Read the model definition and answer for the solid it produces. Units are mm, in the model's axes. A direction names the side the tool comes from. Give positions to 0.01 mm unless a question says otherwise; leave off trailing zeros. Write each loop counter-clockwise with the first axis right and the second up, starting at its lowest first coordinate (ties: lowest second). Pieces come first, ordered by that corner, then holes. Notation, with made-up numbers: M 81.25,25 L 127.25,25 A8 cw 127.25,38 Z; hole C -30.5,14.5 d7. An arc over 180 degrees is marked long. Put each result on its own line as item: value.
from build123d import *

# Parameters (mm, degrees)
SKETCH1_W           = 25.4
SKETCH1_H           = 19.05
SKETCH1_R           = 3.175
SKETCH1_R_2         = 1.016
BOSS_EXTRUDE1_DEPTH = 5
SKETCH1_3_W         = 25.4
SKETCH1_3_H         = 5
BOSS_EXTRUDE2_DEPTH = 20
BOSS_EXTRUDE3_START = 20
SKETCH1_4_W         = 25.4
SKETCH1_4_H         = 19.05
SKETCH1_4_R         = 3.175
SKETCH1_4_R_2       = 1.016
BOSS_EXTRUDE3_DEPTH = 5
SKETCH2_R           = 1.0922
CUT_EXTRUDE1_DEPTH  = 10


with BuildPart() as part:
    # Sketch1 → Boss-Extrude1 (new body)
    with BuildSketch(Plane.XY):
        with Locations((12.7, -9.525)):
            Rectangle(SKETCH1_W, SKETCH1_H)
        with Locations((12.7, -9.525)):
            Circle(SKETCH1_R, mode=Mode.SUBTRACT)
        with Locations((17.4498, -14.2748)):
            Circle(SKETCH1_R_2, mode=Mode.SUBTRACT)
        with Locations((7.9502, -14.2748)):
            Circle(SKETCH1_R_2, mode=Mode.SUBTRACT)
        with Locations((17.4498, -4.7752)):
            Circle(SKETCH1_R_2, mode=Mode.SUBTRACT)
        with Locations((7.9502, -4.7752)):
            Circle(SKETCH1_R_2, mode=Mode.SUBTRACT)
    extrude(amount=BOSS_EXTRUDE1_DEPTH)

    # Sketch1<3> → Boss-Extrude2 (add)
    with BuildSketch(Plane.XY):
        with Locations((12.7, -21.55)):
            Rectangle(SKETCH1_3_W, SKETCH1_3_H)
        Polygon((30.4, 0), (30.4, -24.05), (25.4, -24.05), (25.4, -19.05), (25.4, 0), align=None)
        Polygon((-5, 0), (-5, -24.05), (0, -24.05), (0, -19.05), (0, 0), align=None)
    extrude(amount=BOSS_EXTRUDE2_DEPTH)

    # Sketch1<4> → Boss-Extrude3 (add)
    with BuildSketch(Plane.XY.offset(BOSS_EXTRUDE3_START)):
        with Locations((12.7, -9.525)):
            Rectangle(SKETCH1_4_W, SKETCH1_4_H)
        with Locations((12.7, -9.525)):
            Circle(SKETCH1_4_R, mode=Mode.SUBTRACT)
        with Locations((17.4498, -14.2748)):
            Circle(SKETCH1_4_R_2, mode=Mode.SUBTRACT)
        with Locations((7.9502, -14.2748)):
            Circle(SKETCH1_4_R_2, mode=Mode.SUBTRACT)
        with Locations((17.4498, -4.7752)):
            Circle(SKETCH1_4_R_2, mode=Mode.SUBTRACT)
        with Locations((7.9502, -4.7752)):
            Circle(SKETCH1_4_R_2, mode=Mode.SUBTRACT)
    extrude(amount=-BOSS_EXTRUDE3_DEPTH)

    # Sketch2 → Cut-Extrude1 (cut)
    with BuildSketch(Plane(origin=(0, 0, 0), x_dir=(1, 0, 0), z_dir=(0, 1, 0))):
        with Locations((-2.5, -2.5)):
            Circle(SKETCH2_R)
        with Locations((27.9, -2.5)):
            Circle(SKETCH2_R)
        with Locations((27.9, -17.5)):
            Circle(SKETCH2_R)
        with Locations((-2.5, -17.5)):
            Circle(SKETCH2_R)
    extrude(amount=-CUT_EXTRUDE1_DEPTH, mode=Mode.SUBTRACT)


solid = part.part
(1) Section B-B on y = -18 is taken. Determine the outline of the cut face in (x, z), and give its area (3 significant figures).
Result:
outline: M -5,0 L 30.4,0 L 30.4,20 L -5,20 Z; hole M 0,5 L 25.4,5 L 25.4,15 L 0,15 Z
area: 454 mm²
(2) Section A-A on x = 12.7 is taken. Determine the outline of the cut face in (y, z), and give its area (3 significant figures).
Result:
outline: M -24.05,0 L -12.7,0 L -12.7,5 L -19.05,5 L -19.05,15 L -12.7,15 L -12.7,20 L -24.05,20 Z; M -6.35,0 L 0,0 L 0,5 L -6.35,5 Z; M -6.35,15 L 0,15 L 0,20 L -6.35,20 Z
area: 227 mm²
(3) Section C-C on z = 7.75 is taken. Determine the outline of the cut face in (x, y), and give its area (4 significant figures).
Result:
outline: M -5,-24.05 L 30.4,-24.05 L 30.4,0 L 25.4,0 L 25.4,-19.05 L 0,-19.05 L 0,0 L -5,0 Z
area: 367.5 mm²
(4) For a pull along Z with two mould halves and no side action, classify faces 1 (the face through (12, 0, 3)), 2 (the face through (12, -15, 0)), 3 (the face through (12, -15, 20)), 4 (the face through (28, -10, 17)) as +Z half, -Z half, draft (parallel to the pull), parting line (faces both ways), or undercut.
Result:
face 1: draft
face 2: -Z half
face 3: +Z half
face 4: undercut
(5) Straight lines are drawn through the part: line 1 along Z through (x, y) = (22, -8); line 2 along X through (y, z) = (-2, 2.5); line 3 along Y through (x, z) = (12.7, 1.1). For each, find the intervals that lie inside material, in ascending order. Write a range as from..to.
Result:
line 1: z = 0..5, 15..20
line 2: x = -5..-3.59, -1.41..26.81, 28.99..30.4
line 3: y = -24.05..-12.7, -6.35..0
(6) Given pin 1 Ø1.2 at (x, y) = (17.45, -14.27) entering from +Z; pin 2 Ø0.7 at (x, z) = (-2, 17.5) entering from +Y, each flat-ended and moving along its own axis, determine where each tip first touches the part or whether it passes through.
Result:
pin 1: passes through
pin 2: stops at y = -10
(7) Section D-D on y = -6.75 is taken. Determine the outline of the cut face in (x, z).
Result:
outline: M -5,0 L 11.16,0 L 11.16,5 L 0,5 L 0,15 L 11.16,15 L 11.16,20 L -5,20 Z; M 14.24,0 L 30.4,0 L 30.4,20 L 14.24,20 L 14.24,15 L 25.4,15 L 25.4,5 L 14.24,5 Z; hole C -2.5,2.5 d2.18; hole C -2.5,17.5 d2.18; hole C 27.9,2.5 d2.18; hole C 27.9,17.5 d2.18
(8) Which of the six approach directions +Z, -Z, +X, -X, +Y, -Y give full straight-line access (tool end or side, diameter ignored) to faces 5 (the face through (12, -24.05, 10)), 6 (the face through (-3, -10, 2))?
Result:
face 5: +Z, -Z, +X, -X, -Y
face 6: +Y
